```python
from build123d import *

# Parameters (mm, degrees)
F0_W     = 20
F0_H     = 20
F1_DEPTH = 20
F2_R     = 2.6
F3_DEPTH = 1
F4_R     = 2.6
F5_DEPTH = 1


with BuildPart() as f1:
    # F0 (on Front) → F1 (new body)
    with BuildSketch(Plane.XZ):
        with Locations((-10, 10)):
            Rectangle(F0_W, F0_H)
    extrude(amount=F1_DEPTH)

    # F2 (on face) → F3 (cut)
    with BuildSketch(Plane(origin=(0, 0, 0), x_dir=(-1, 0, 0), z_dir=(0, 1, 0))):
        with Locations((10, 10)):
            Circle(F2_R)
        with Locations((5, 15)):
            Circle(F2_R)
        with Locations((5, 5)):
            Circle(F2_R)
        with Locations((15, 15)):
            Circle(F2_R)
        with Locations((15, 5)):
            Circle(F2_R)
    extrude(amount=-F3_DEPTH, mode=Mode.SUBTRACT)

    # F4 (on face) → F5 (join)
    with BuildSketch(Plane.XZ.offset(20)):
        with Locations((-5, 15)):
            Circle(F4_R)
        with Locations((-15, 5)):
            Circle(F4_R)
    extrude(amount=F5_DEPTH)


solid = f1.part
```
Geometry: final body of the model. Coordinates: model frame, mm. A direction names the side the tool comes from. Coordinates: 2 decimals unless noted, no trailing zeros. Order: outer loops, then holes, each group sorted by start corner. A loop starts at its lowest first (then second) coordinate and runs counter-clockwise, first axis right, second up. Notation, with made-up numbers: (33, 16) - (57, 16) arc R21 ccw to (57, 34) - close; hole circle Ø4 at (-21.75, 41.5). An arc over 180 degrees is marked (long way). Return JSON: item names as keys, results as strings. Group by question number.
1. Material intervals for line 1 along Z through (x, y) = (-5, -0.5); line 2 along Z through (x, y) = (-10, -0.45); line 3 along Y through (x, z) = (-8.75, 6.75), sorted ascending. Write a range as [from, to].
2. Cut plane A-A (x = -10). Output: boundary loops of the cut face in (y, z).
3. Pin query (flat end, axial travel): pin 1 (4.5 mm diameter, centred on x = -5, z = 5, fed in from +Y); pin 2 (7 mm diameter, centred on x = -10, z = 10, fed in from -Y). Return the tip coordinate at first contact, or that it passes through.
4. Cut plane D-D (x = -3). Output: boundary loops of the cut face in (y, z).
5. Cut plane C-C (z = 11.25). Output: boundary loops of the cut face in (x, y).
6. Set-up query: faces 4 (the face through (-5, -1, 15)), 5 (the face through (-3.8, -20.493, 12.693)), 6 (the face through (-8, 0, 8)). Return all of +Z, -Z, +X, -X, +Y, -Y with unobstructed straight access to the full face (end or side cutting, diameter ignored); none if empty.
7. Pull-direction query (X, two-part tool) for faces 1 (the face through (-10, -20, 10)), 2 (the face through (-15, -1, 5)), 3 (the face through (-12.52, -20.49, 5.78)); classes: pulls with the +X half, pulls with the -X half, needs draft (parallel to the pull), parting line crosses it, or undercut.
8. Cut plane B-B (z = 15). Output: boundary loops of the cut face in (x, y).
Resolved:
{
 "1": {"line 1": "z = [0, 2.4], [7.6, 12.4], [17.6, 20]", "line 2": "z = [0, 7.4], [12.6, 20]", "line 3": "y = [-20, 0]"},
 "2": {"outline": "(-20, 0) - (0, 0) - (0, 7.4) - (-1, 7.4) - (-1, 12.6) - (0, 12.6) - (0, 20) - (-20, 20) - close"},
 "3": {"pin 1": "stops at y = -1", "pin 2": "stops at y = -20"},
 "4": {"outline": "(-21, 13.34) - (-20, 13.34) - (-20, 0) - (0, 0) - (0, 3.34) - (-1, 3.34) - (-1, 6.66) - (0, 6.66) - (0, 13.34) - (-1, 13.34) - (-1, 16.66) - (0, 16.66) - (0, 20) - (-20, 20) - (-20, 16.66) - (-21, 16.66) - close"},
 "5": {"outline": "(-20, -20) - (0, -20) - (0, 0) - (-7.72, 0) - (-7.72, -1) - (-12.28, -1) - (-12.28, 0) - (-20, 0) - close"},
 "6": {"face 4": "+Y", "face 5": "-Y", "face 6": "+Z, -Z, +X, -X, +Y"},
 "7": {"face 1": "needs draft", "face 2": "undercut", "face 3": "parting line crosses it"},
 "8": {"outline": "(-20, -20) - (-7.6, -20) - (-7.6, -21) - (-2.4, -21) - (-2.4, -20) - (0, -20) - (0, 0) - (-2.4, 0) - (-2.4, -1) - (-7.6, -1) - (-7.6, 0) - (-12.4, 0) - (-12.4, -1) - (-17.6, -1) - (-17.6, 0) - (-20, 0) - close"}
}
